Design review of the part shown in the three views and the two pictorial views. Dimensions are in mm from the part's minimum x, y and z. A direction names the side the tool comes from. Give positions to 0.01 mm unless a question says otherwise; leave off trailing zeros. Loops run counter-clockwise (first coordinate to the right, second up) from the corner with the lowest first, then second, coordinate; pieces in that order, holes last. Notation, with made-up numbers: (-36, 4.5) -> (-7, 4.5) arc R16 ccw to (-7, 21.5) -> close; hole circle Ø6 at (-19, 59). An arc over 180 degrees is marked (long way). One line per question, with ' | ' between items. Start each with the question number.
(1) Insertion check: P1, Ø15, axis at x = 25.5, y = 22, coming from the +Z side; P2, Ø4, axis at x = 4.5, y = 4, coming from the +Z side; P3, Ø1, axis at x = 25.5, y = 12, coming from the -Z side. Each pin has a flat end and moves straight along its axis. Give the tip position at first contact, or say it passes through.
(2) Consider section C-C (x = 45.25). Write out the cut boundary in (y, z).
(3) Tool access review of the marked faces 1, 2 and 3: name each direction out of +Z, -Z, +X, -X, +Y, -Y from which nothing blocks a thin tool from reaching the whole face with its end or side.
(4) Wall thickness on probe 1 along X at (y, z) = (28.75, 2.55); probe 2 along X at (y, z) = (3.75, 1.1); probe 3 along Y at (x, z) = (45.25, 1.45): over which ranges is each line inside the solid? List them lowest first.
(5) Consider section B-B (y = 14). Write out the cut boundary in (x, z).
(6) Consider section D-D (z = 6.5). Write out the cut boundary in (x, y), and give its area (3 significant figures).
(7) Draft analysis for pull direction Y (two halves, no side actions). For the marked faces 4, 5, 6 and 7, state which applies: +Y half, -Y half, draft (parallel to the pull), parting line (faces both ways), or undercut.
(8) Consider section A-A (x = 3.75). Write out the cut boundary in (y, z), and give its area (3 significant figures).
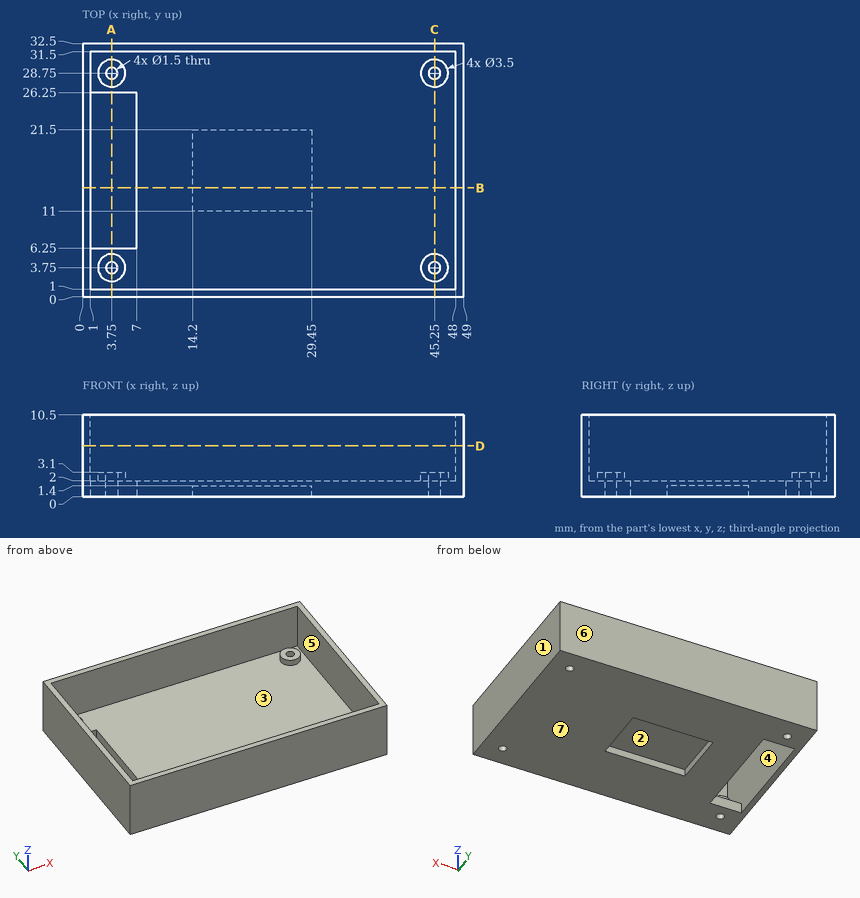
A:
1) P1: stops at z = 2 | P2: stops at z = 3.1 | P3: stops at z = 1.4
2) outline: (0, 0) -> (3, 0) -> (3, 3.1) -> (2, 3.1) -> (2, 2) -> (1, 2) -> (1, 10.5) -> (0, 10.5) -> close; (4.5, 0) -> (28, 0) -> (28, 3.1) -> (27, 3.1) -> (27, 2) -> (5.5, 2) -> (5.5, 3.1) -> (4.5, 3.1) -> close; (29.5, 0) -> (32.5, 0) -> (32.5, 10.5) -> (31.5, 10.5) -> (31.5, 2) -> (30.5, 2) -> (30.5, 3.1) -> (29.5, 3.1) -> close
3) face 1: +Z, -Z, +X, +Y, -Y | face 2: -Z | face 3: +Z
4) probe 1: x = 0 to 1, 2 to 3, 4.5 to 5.5, 43.5 to 44.5, 46 to 47, 48 to 49 | probe 2: x = 0 to 3, 4.5 to 44.5, 46 to 49 | probe 3: y = 0 to 3, 4.5 to 28, 29.5 to 32.5
5) outline: (0, 0) -> (1, 0) -> (1, 10.5) -> (0, 10.5) -> close; (7, 0) -> (14.2, 0) -> (14.2, 1.4) -> (29.45, 1.4) -> (29.45, 0) -> (49, 0) -> (49, 10.5) -> (48, 10.5) -> (48, 2) -> (7, 2) -> close
6) outline: (0, 0) -> (49, 0) -> (49, 32.5) -> (0, 32.5) -> close; hole (1, 1) -> (48, 1) -> (48, 31.5) -> (1, 31.5) -> close | area: 159 mm^2
7) face 4: undercut | face 5: undercut | face 6: +Y half | face 7: draft
8) outline: (0, 0) -> (3, 0) -> (3, 3.1) -> (2, 3.1) -> (2, 2) -> (1, 2) -> (1, 10.5) -> (0, 10.5) -> close; (4.5, 0) -> (6.25, 0) -> (6.25, 2) -> (5.5, 2) -> (5.5, 3.1) -> (4.5, 3.1) -> close; (26.25, 0) -> (28, 0) -> (28, 3.1) -> (27, 3.1) -> (27, 2) -> (26.25, 2) -> close; (29.5, 0) -> (32.5, 0) -> (32.5, 10.5) -> (31.5, 10.5) -> (31.5, 2) -> (30.5, 2) -> (30.5, 3.1) -> (29.5, 3.1) -> close | area: 40.4 mm^2
